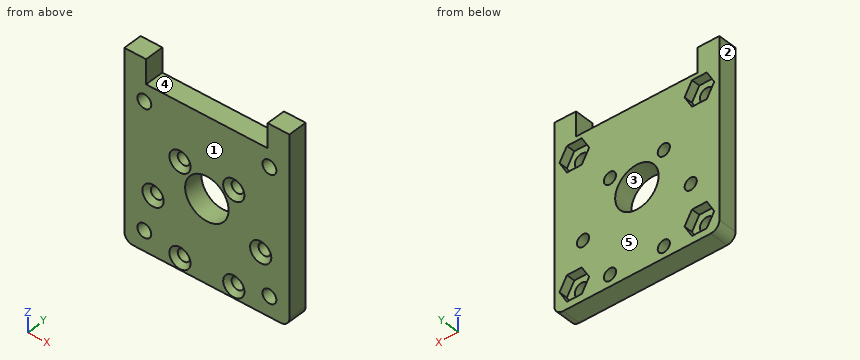
```python
from build123d import *

# Parameters (mm, degrees)
SKETCH_R     = 6.25
SKETCH_R_2   = 1.75
SKETCH_R_3   = 2
PAD_DEPTH    = 5.5
CHAMFER_SIZE = 1.3
POCKET_DEPTH = 2.5


with BuildPart() as part:
    # Sketch → Pad (new body)
    with BuildSketch(Plane.XZ):
        with BuildLine():
            Line((21.25, -16.75), (-21.25, -16.75))
            ThreePointArc((-23.75, -14.25), (-23.017767, -16.017767), (-21.25, -16.75))
            Line((-23.75, 37), (-23.75, -14.25))
            Line((-23.75, 37), (-17.5, 37))
            Line((-17.5, 37), (-17.5, 30))
            Line((-17.5, 30), (17.5, 30))
            Line((17.5, 30), (17.5, 37))
            Line((17.5, 37), (23.75, 37))
            Line((23.75, 37), (23.75, -14.25))
            ThreePointArc((21.25, -16.75), (23.017767, -16.017767), (23.75, -14.25))
        make_face()
        with Locations((0, 7)):
            Circle(SKETCH_R, mode=Mode.SUBTRACT)
        with Locations((-7.75, 13.423394)):
            Circle(SKETCH_R_2, mode=Mode.SUBTRACT)
        with Locations((-15.5, 0)):
            Circle(SKETCH_R_2, mode=Mode.SUBTRACT)
        with Locations((-7.75, -13.423394)):
            Circle(SKETCH_R_2, mode=Mode.SUBTRACT)
        with Locations((7.75, -13.423394)):
            Circle(SKETCH_R_2, mode=Mode.SUBTRACT)
        with Locations((15.5, 0)):
            Circle(SKETCH_R_2, mode=Mode.SUBTRACT)
        with Locations((7.75, 13.423394)):
            Circle(SKETCH_R_2, mode=Mode.SUBTRACT)
        with Locations((-18, 25)):
            Circle(SKETCH_R_3, mode=Mode.SUBTRACT)
        with Locations((18, 25)):
            Circle(SKETCH_R_3, mode=Mode.SUBTRACT)
        with Locations((18, -11)):
            Circle(SKETCH_R_3, mode=Mode.SUBTRACT)
        with Locations((-18, -11)):
            Circle(SKETCH_R_3, mode=Mode.SUBTRACT)
    extrude(amount=PAD_DEPTH)

    # Chamfer
    chamfer_edges = [part.edges().sort_by_distance(p)[0] for p in [
        (-9.5, -5.5, 13.423394),
        (13.75, -5.5, 0),
        (6, -5.5, 13.423394),
        (-17.25, -5.5, 0),
        (6, -5.5, -13.423394),
        (-9.5, -5.5, -13.423394),
    ]]
    chamfer(chamfer_edges, length=CHAMFER_SIZE)

    # Sketch001 → Pocket (cut)
    with BuildSketch(Plane.XZ):
        Polygon((-15.863804, 28.7), (-20.136196, 28.7), (-22.272392, 25), (-20.136196, 21.3), (-15.863804, 21.3), (-13.727608, 25), align=None)
        Polygon((20.136196, 28.7), (15.863804, 28.7), (13.727608, 25), (15.863804, 21.3), (20.136196, 21.3), (22.272392, 25), align=None)
        Polygon((20.136196, -7.3), (15.863804, -7.3), (13.727608, -11), (15.863804, -14.7), (20.136196, -14.7), (22.272392, -11), align=None)
        Polygon((-15.863804, -7.3), (-20.136196, -7.3), (-22.272392, -11), (-20.136196, -14.7), (-15.863804, -14.7), (-13.727608, -11), align=None)
    extrude(amount=POCKET_DEPTH, mode=Mode.SUBTRACT)


solid = part.part
```
Check sheet for the modelled part. Datum: model origin and axes. Units: mm. Face numbers are marked on the shaded views. A direction names the side the tool comes from. Round coordinates to 2 decimals unless told otherwise and drop trailing zeros. Order: outer loops, then holes, each group sorted by start corner. A loop starts at its lowest first (then second) coordinate and runs counter-clockwise, first axis right, second up. Notation, with made-up numbers: (10.5, -5.75) -> (36.5, -5.75) arc R33 ccw to (36.5, 24.25) -> close; hole circle Ø9 at (58, -26.75). An arc over 180 degrees is marked (long way). Use CSV: the item, a comma, the result in double quotes.
(1) Cross-section at B-B (z = 7). Record the boundary of the cut face in (x, y).
Worked out:
outline,"(-23.75, -5.5) -> (-6.25, -5.5) -> (-6.25, 0) -> (-23.75, 0) -> close; (6.25, -5.5) -> (23.75, -5.5) -> (23.75, 0) -> (6.25, 0) -> close"
(2) Cross-section at A-A (z = 0). Record the boundary of the cut face in (x, y), and give its area (3 significant figures).
Worked out:
outline,"(-23.75, -5.5) -> (-18.55, -5.5) -> (-17.25, -4.2) -> (-17.25, 0) -> (-23.75, 0) -> close; (-13.75, -4.2) -> (-12.45, -5.5) -> (12.45, -5.5) -> (13.75, -4.2) -> (13.75, 0) -> (-13.75, 0) -> close; (17.25, -4.2) -> (18.55, -5.5) -> (23.75, -5.5) -> (23.75, 0) -> (17.25, 0) -> close"
area,"219 mm²"
(3) Cross-section at C-C (y = -3.4). Count the separate pieces of the cut face and the enclosed holes in it, and give its area (3 significant figures).
Worked out:
separate pieces,"1"
enclosed holes,"11"
area,"2,070 mm²"
(4) Draft check along X on the marked faces 1, 2 and 3. Enter one of: pulls with the +X half, pulls with the -X half, needs draft (parallel to the pull), parting line crosses it, or undercut.
Worked out:
face 1,"needs draft"
face 2,"pulls with the -X half"
face 3,"undercut"
(5) Depth check by flat-ended pin: pin 1 (3 mm diameter, centred on x = 7.75, z = 13.42, fed in from +Y); pin 2 (4.5 mm diameter, centred on x = -18, z = -11, fed in from +Y); pin 3 (4 mm diameter, centred on x = -7.75, z = -13.42, fed in from -Y). Enter the tip coordinate at first touch or a pass-through.
Worked out:
pin 1,"through"
pin 2,"y = -2.5"
pin 3,"y = -4.45"
(6) Material ranges on line 1 along Z through (x, y) = (7.75, -2.5); line 2 along Z through (x, y) = (-18.5, -1.75); line 3 along X through (y, z) = (-4.5, 25), recorded low to high. Write a range as from..to.
Worked out:
line 1,"-16.75..-15.17, -11.67..11.67, 15.17..30"
line 2,"-16.75..-14.7, -7.3..21.3, 28.7..37"
line 3,"-23.75..-20, -16..16, 20..23.75"
(7) Tool access check on the marked faces 4 and 5. Record the directions out of +Z, -Z, +X, -X, +Y, -Y that give a thin tool (end or side, any length) a straight path to the whole face; none if there is none.
Worked out:
face 4,"+Z, +Y, -Y"
face 5,"+Z, -Z, +X, -X, +Y"
